Check sheet for the modelled part. Datum: model origin and axes. Units: mm. Face numbers are marked on the shaded views. A direction names the side the tool comes from. Round coordinates to 2 decimals unless told otherwise and drop trailing zeros. Answer in a Markdown table with one row per item.
from build123d import *

# Parameters (mm, degrees)
CHAMFER1_SIZE = 0.396875
FILLET1_R     = 0.1905
FILLET2_R     = 0.127
CHAMFER2_SIZE = 0.3175


with BuildPart() as part:
    # Sketch3 → Revolve1 (revolve)
    with BuildSketch(Plane(origin=(0, 0, 0), x_dir=(0, 0, -1), z_dir=(1, 0, 0)), mode=Mode.PRIVATE) as revolve1_sk:
        Polygon((-4.7625, 3.175), (4.7625, 3.175), (4.7625, 6.35), (3.175, 6.35), (3.175, 4.7625), (-4.7625, 4.7625), align=None)
    revolve(revolve1_sk.sketch.rotate(Axis((0, 0, 4.7625), (0, 0, -1)), 180), axis=Axis((0, 0, 4.7625), (0, 0, -1)))

    # Chamfer1
    chamfer1_edges = [part.edges().sort_by_distance(p)[0] for p in [
        (0, 4.7625, 4.7625),
    ]]
    chamfer(chamfer1_edges, length=CHAMFER1_SIZE)

    # Fillet1
    fillet1_edges = [part.edges().sort_by_distance(p)[0] for p in [
        (0, 4.7625, -3.175),
    ]]
    fillet(fillet1_edges, radius=FILLET1_R)

    # Fillet2
    fillet2_edges = [part.edges().sort_by_distance(p)[0] for p in [
        (0, 6.35, -3.175),
        (0, 6.35, -4.7625),
    ]]
    fillet(fillet2_edges, radius=FILLET2_R)

    # Chamfer2
    chamfer2_edges = [part.edges().sort_by_distance(p)[0] for p in [
        (0, 3.175, -4.7625),
    ]]
    chamfer(chamfer2_edges, length=CHAMFER2_SIZE)


solid = part.part
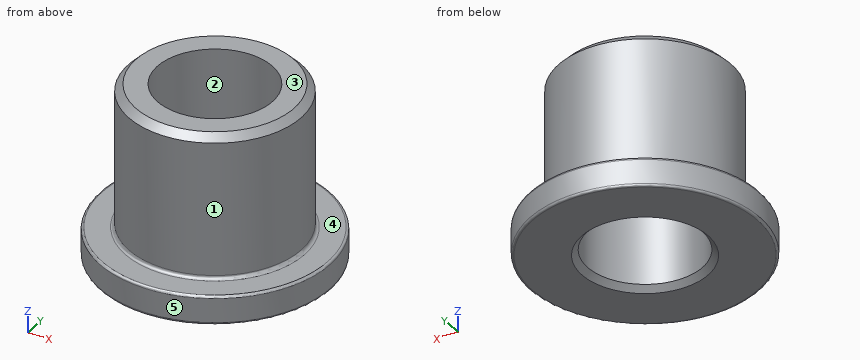
Item 1: Scan lines: line 1 (X direction, y = 0, z = -0.75) (1 decimal); line 2 (X direction, y = 0.5, z = 2); line 3 (Y direction, x = 2, z = -3). Record each from-to range of solid material in increasing order. Write a range as [from, to].
Result sheet:
| item | result |
|---|---|
| line 1 | x = [-4.8, -3.2], [3.2, 4.8] |
| line 2 | x = [-4.74, -3.14], [3.14, 4.74] |
| line 3 | y = [-4.32, -2.47], [2.47, 4.32] |
Item 2: Depth check by flat-ended pin: P1, Ø5, axis at y = 2, z = -0.5, coming from the -X side; P2, Ø2, axis at x = -1.5, z = -2, coming from the +Y side; P3, Ø1.5, axis at y = 0, z = -2, coming from the +X side. Enter the tip coordinate at first touch or a pass-through.
Result sheet:
| item | result |
|---|---|
| P1 | stops at x = -4.76 |
| P2 | stops at y = 4.74 |
| P3 | stops at x = 4.76 |
Item 3: Mould release check, pull along X, two halves, no side actions. Record for the marked faces 1, 2 and 3: pulls with the +X half, pulls with the -X half, needs draft (parallel to the pull), parting line crosses it, or undercut.
Result sheet:
| item | result |
|---|---|
| face 1 | parting line crosses it |
| face 2 | undercut |
| face 3 | needs draft |
Item 4: Set-up check for the marked faces 4 and 5: record each of +Z, -Z, +X, -X, +Y, -Y from which the full face is reachable in a straight line by a thin tool's end or side.
Result sheet:
| item | result |
|---|---|
| face 4 | +Z |
| face 5 | +Z, -Z |
